Check sheet for the drawn part. Datum: minimum x, y, z corner. Units: mm. A direction names the side the tool comes from. Coordinates: 2 decimals unless noted, no trailing zeros. Loops run counter-clockwise (first coordinate to the right, second up) from the corner with the lowest first, then second, coordinate; pieces in that order, holes last.
Q1. Access from +Z, -Z, +X, -X, +Y, -Y to the whole of each face (thin tool, end or side, straight path). Record for the marked faces 4 and 5.
Q2. Material ranges on probe 1 along Y at (x, z) = (37.5, 47); probe 2 along X at (y, z) = (37, 140), recorded low to high.
Q3. Go/stop test with flat-tipped pins: P1, Ø10, axis at x = 13.5, y = 37.5, coming from the +Z side; P2, Ø10, axis at x = 11, z = 41, coming from the -Y side. Record where each tip stops, or that it passes through.
Q4. Sectioned sample at B-B (y = 26.5). Enter the section's corners in (x, z), then the cut area to 3 significant figures.
Q5. Sectioned sample at A-A (z = 112). Enter the section's corners in (x, y).
Q6. Sectioned sample at C-C (x = 42.5). Enter the section's corners in (y, z).
Q7. Mould release check, pull along X, two halves, no side actions. Record for the marked faces 1, 2 and 3: +X half, -X half, draft (parallel to the pull), parting line (faces both ways), or undercut.
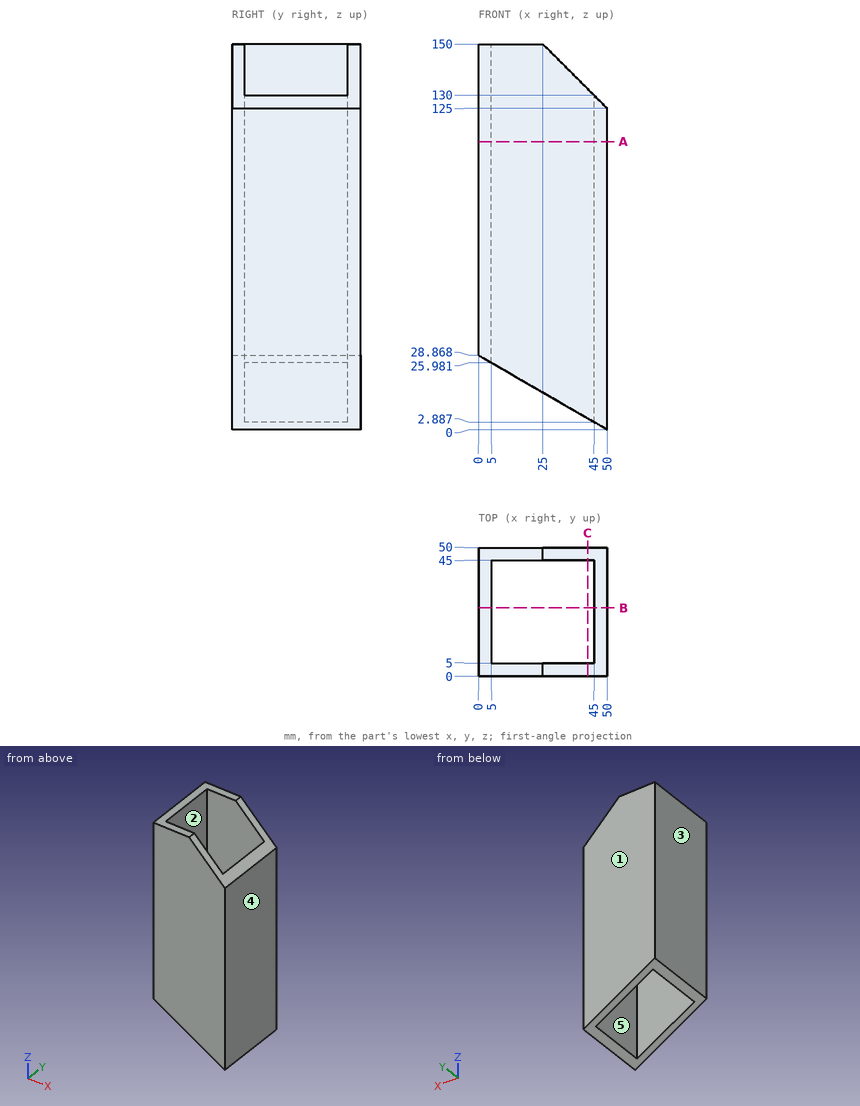
Geometry check:
1. face 4: +Z, -Z, +X, +Y, -Y
1. face 5: +Z, -Z
2. probe 1: y = 0 to 5, 45 to 50
2. probe 2: x = 0 to 5
3. P1: passes through
3. P2: stops at y = 0
4. outline: (0, 28.87) - (5, 25.98) - (5, 150) - (0, 150) - close; (45, 2.89) - (50, 0) - (50, 125) - (45, 130) - close
4. area: 1,240 mm2
5. outline: (0, 0) - (50, 0) - (50, 50) - (0, 50) - close; hole (5, 5) - (45, 5) - (45, 45) - (5, 45) - close
6. outline: (0, 4.33) - (5, 4.33) - (5, 132.5) - (0, 132.5) - close; (45, 4.33) - (50, 4.33) - (50, 132.5) - (45, 132.5) - close
7. face 1: draft
7. face 2: undercut
7. face 3: -X half
